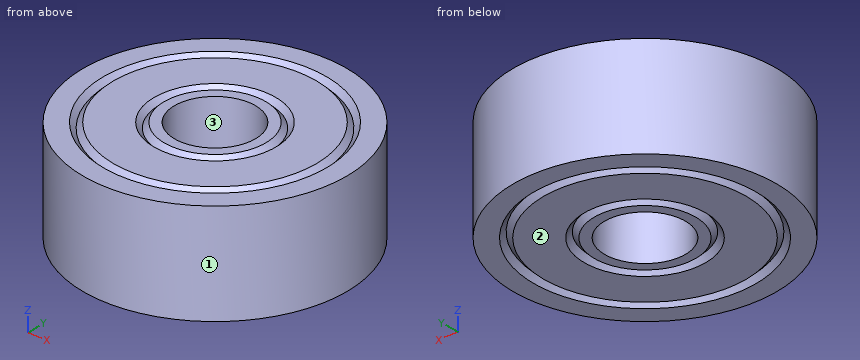
from build123d import *

# Parameters (mm, degrees)
SKETCH1_R           = 6.5
SKETCH1_R_2         = 2
BOSS_EXTRUDE1_DEPTH = 5


with BuildPart() as part:
    # Sketch1 → Boss-Extrude1 (new body)
    with BuildSketch(Plane.XY):
        Circle(SKETCH1_R)
        Circle(SKETCH1_R_2, mode=Mode.SUBTRACT)
    extrude(amount=BOSS_EXTRUDE1_DEPTH)

    # Sketch2 → Cut-Revolve1 (revolve, cut)
    with BuildSketch(Plane(origin=(0, 0, 0), x_dir=(0, 0, -1), z_dir=(1, 0, 0)), mode=Mode.PRIVATE) as cut_revolve1_sk:
        Polygon((-5, 5.5), (-5, 5), (-4.75, 5.25), align=None)
        Polygon((-5, 3), (-5, 2.5), (-4.75, 2.75), align=None)
        Polygon((-0.25, 2.75), (0, 3), (0, 2.5), align=None)
        Polygon((-0.25, 5.25), (0, 5.5), (0, 5), align=None)
    revolve(cut_revolve1_sk.sketch.rotate(Axis((0, 0, 0), (0, 0, 1)), 90), axis=Axis((0, 0, 0), (0, 0, 1)), mode=Mode.SUBTRACT)


solid = part.part
Check sheet for the modelled part. Datum: model origin and axes. Units: mm. Face numbers are marked on the shaded views. Coordinates: 2 decimals unless noted, no trailing zeros. Loops run counter-clockwise (first coordinate to the right, second up) from the corner with the lowest first, then second, coordinate; pieces in that order, holes last. Notation, with made-up numbers: (0.25, 9.5) -> (58.25, 9.5) arc R24 ccw to (58.25, 37.5) -> close; hole circle Ø11 at (77, 16). An arc over 180 degrees is marked (long way). Write item = value, one per line. Start each with the question number.
1. Depth check by flat-ended pin: P1, Ø1.5, axis at y = -1, z = 2.5, coming from the -X side; P2, Ø3, axis at x = 0, y = 0, coming from the +Z side; P3, Ø3, axis at x = -2, z = 2.5, coming from the -Y side; P4, Ø1.5, axis at y = 3.5, z = 1, coming from the +X side. Enter the tip coordinate at first touch or a pass-through.
2. Material ranges on line 1 (Y direction, x = 0, z = 3.05); line 2 (Y direction, x = -0.5, z = 1.8); line 3 (X direction, y = 1, z = 4.35), recorded low to high.
3. Draft check along X on the marked faces 1, 2 and 3. Enter one of: released by +X, released by -X, zero draft, split by the parting line, or undercut.
4. Section check C-C on z = 4.3. Record the cut outline in (x, y), then the cut area to 3 significant figures.
Responses:
q1.P1 = -6.5
q1.P2 = through
q1.P3 = -6.48
q1.P4 = 5.89
q2.line_1 = -6.5 to -2, 2 to 6.5
q2.line_2 = -6.48 to -1.94, 1.94 to 6.48
q2.line_3 = -6.42 to -1.73, 1.73 to 6.42
q3.face_1 = split by the parting line
q3.face_2 = zero draft
q3.face_3 = undercut
q4.outline = circle Ø13 at (0, 0); hole circle Ø4 at (0, 0)
q4.area = 120 mm2
